```python
from build123d import *

# Parameters (mm, degrees)
SKETCH1_W                 = 55.88
SKETCH1_H                 = 6.35
CUT_EXTRUDE1_START        = -5.588
CUT_EXTRUDE1_DEPTH        = 5.588
CUT_EXTRUDE2_DEPTH        = 5.588
F_8_32_TAPPED_HOLE1_D     = 3.4544
F_8_32_TAPPED_HOLE1_DEPTH = 12.7
F_8_32_TAPPED_HOLE1_TIP   = 1.037806461
F_8_32_TAPPED_HOLE2_D     = 3.4544
F_8_32_TAPPED_HOLE2_DEPTH = 12.7
F_8_32_TAPPED_HOLE2_TIP   = 1.037806461
FILLET1_R                 = 1.5875
CHAMFER1_SIZE             = 0.254
CUT_EXTRUDE3_DEPTH        = 1.5875


with BuildPart() as part:
    # Sketch1 → Revolve1 (revolve)
    with BuildSketch(Plane(origin=(0, 0, 0), x_dir=(0, 0, -1), z_dir=(1, 0, 0)), mode=Mode.PRIVATE) as revolve1_sk:
        with Locations((27.94, 3.175)):
            Rectangle(SKETCH1_W, SKETCH1_H)
    revolve(revolve1_sk.sketch.rotate(Axis((0, 0, 0), (0, 0, -1)), 90), axis=Axis((0, 0, 0), (0, 0, -1)))

    # Sketch5 → Cut-Extrude1 (cut)
    with BuildSketch(Plane.XY.offset(CUT_EXTRUDE1_START)):
        with BuildLine():
            Line((-4.200130206, 4.7625), (4.200130206, 4.7625))
            ThreePointArc((4.200130206, 4.7625), (0, 6.35), (-4.200130206, 4.7625))
        make_face()
        with BuildLine():
            Line((-4.200130206, -4.7625), (4.200130206, -4.7625))
            ThreePointArc((4.200130206, -4.7625), (0, -6.35), (-4.200130206, -4.7625))
        make_face()
    extrude(amount=CUT_EXTRUDE1_DEPTH, mode=Mode.SUBTRACT)

    # Sketch6 → Cut-Extrude2 (cut)
    with BuildSketch(Plane(origin=(0, 0, -55.88), x_dir=(-1, 0, 0), z_dir=(0, 0, -1))):
        with BuildLine():
            Line((-4.200130206, 4.7625), (4.200130206, 4.7625))
            ThreePointArc((4.200130206, 4.7625), (0, 6.35), (-4.200130206, 4.7625))
        make_face()
        with BuildLine():
            Line((4.200130206, -4.7625), (-4.200130206, -4.7625))
            ThreePointArc((-4.200130206, -4.7625), (0, -6.35), (4.200130206, -4.7625))
        make_face()
    extrude(amount=-CUT_EXTRUDE2_DEPTH, mode=Mode.SUBTRACT)

    # #8-32 Tapped Hole1
    with Locations(Plane.XY):
        with Locations((0, 0)):
            Hole(F_8_32_TAPPED_HOLE1_D / 2, depth=F_8_32_TAPPED_HOLE1_DEPTH)
            with Locations((0, 0, -(F_8_32_TAPPED_HOLE1_DEPTH + F_8_32_TAPPED_HOLE1_TIP / 2))):  # 118° drill point
                Cone(0, F_8_32_TAPPED_HOLE1_D / 2, F_8_32_TAPPED_HOLE1_TIP, mode=Mode.SUBTRACT)

    # #8-32 Tapped Hole2
    with Locations(Plane(origin=(0, 0, -55.88), x_dir=(-1, 0, 0), z_dir=(0, 0, -1))):
        with Locations((0, 0)):
            Hole(F_8_32_TAPPED_HOLE2_D / 2, depth=F_8_32_TAPPED_HOLE2_DEPTH)
            with Locations((0, 0, -(F_8_32_TAPPED_HOLE2_DEPTH + F_8_32_TAPPED_HOLE2_TIP / 2))):  # 118° drill point
                Cone(0, F_8_32_TAPPED_HOLE2_D / 2, F_8_32_TAPPED_HOLE2_TIP, mode=Mode.SUBTRACT)

    # Fillet1
    fillet1_edges = [part.edges().sort_by_distance(p)[0] for p in [
        (-4.200130206, 4.7625, -2.794),
        (4.200130206, 4.7625, -2.794),
        (4.200130206, -4.7625, -2.794),
        (-4.200130206, -4.7625, -2.794),
        (4.200130206, 4.7625, -53.086),
        (-4.200130206, 4.7625, -53.086),
        (-4.200130206, -4.7625, -53.086),
        (4.200130206, -4.7625, -53.086),
    ]]
    fillet(fillet1_edges, radius=FILLET1_R)

    # Chamfer1
    chamfer1_edges = [part.edges().sort_by_distance(p)[0] for p in [
        (-6.35, 0, -55.88),
        (5.931994479, -2.26582027, -55.88),
        (-6.35, 0, 0),
        (5.931994479, -2.26582027, 0),
        (0, -4.7625, 0),
        (0, 4.7625, 0),
        (-4.197852075, 4.6241826, 0),
        (4.197852075, 4.6241826, 0),
        (4.197852075, -4.6241826, 0),
        (-4.197852075, -4.6241826, 0),
        (0, -4.7625, -55.88),
        (0, 4.7625, -55.88),
        (4.197852075, 4.6241826, -55.88),
        (-4.197852075, 4.6241826, -55.88),
        (4.197852075, -4.6241826, -55.88),
        (-4.197852075, -4.6241826, -55.88),
    ]]
    chamfer(chamfer1_edges, length=CHAMFER1_SIZE)

    # Sketch11 → Cut-Extrude3 (cut)
    with BuildSketch(Plane(origin=(0, 6.35, 0), x_dir=(-1, 0, 0), z_dir=(0, 1, 0))):
        with BuildLine():
            Line((-1.5875, -34.29), (-1.5875, -21.59))
            ThreePointArc((-1.5875, -21.59), (0, -20.0025), (1.5875, -21.59))
            Line((1.5875, -21.59), (1.5875, -34.29))
            ThreePointArc((1.5875, -34.29), (0, -35.8775), (-1.5875, -34.29))
        make_face()
    extrude(amount=-CUT_EXTRUDE3_DEPTH, mode=Mode.SUBTRACT)


solid = part.part
```
The listing builds one solid part. Answer for the finished solid, in the listing's coordinates (mm). A direction names the side the tool comes from. Give positions to 0.01 mm unless a question says otherwise; leave off trailing zeros. Loops run counter-clockwise (first coordinate to the right, second up) from the corner with the lowest first, then second, coordinate; pieces in that order, holes last. Notation, with made-up numbers: M 58,-12 L 77,-12 A37 ccw 77,26 Z; hole C -19.5,72.25 d5. An arc over 180 degrees is marked long. One line per item, written item: value.
1. Find the intervals of material crossed by probe 1 along Y at (x, z) = (0, -4.5); probe 2 along Y at (x, z) = (0, -45.5); probe 3 along Z at (x, y) = (-1.75, 5.5), in increasing order.
Found:
probe 1: -4.76 to -1.73, 1.73 to 4.76
probe 2: -6.35 to -1.73, 1.73 to 6.35
probe 3: -50.29 to -5.59
2. For a pull along Y with two mould halves and no side action, classify faces 4 (the face through (-0.225, 1.713, -49.441)), 5 (the face through (1.588, 5, -28)), 6 (the face through (-0.138, -0.266, -42.322)), 7 (the face through (-4.21, -4.62, -2.88)) as pulls with the +Y half, pulls with the -Y half, needs draft (parallel to the pull), parting line crosses it, or undercut.
Found:
face 4: undercut
face 5: needs draft
face 6: undercut
face 7: pulls with the -Y half
3. Each of these flat-tipped pins is pushed along its axis until it touches: P1, Ø2, axis at x = 0, y = 0, coming from the -Z side; P2, Ø2, axis at x = 1.5, z = -23.5, coming from the -Y side; P3, Ø2.5, axis at x = 0, z = -26, coming from the +Y side. Where does it stop, or does it pass through?
Found:
P1: z = -42.74
P2: y = -6.33
P3: y = 4.76
4. For faces 1 (the face through (-0.035, 5.568, -35.877)), 2 (the face through (0, -4.762, -53)), 3 (the face through (-4.21, 4.62, -52.92)), determine the directions among +Z, -Z, +X, -X, +Y, -Y from which every point of the face is accessible in a straight line to the end or side of a thin tool.
Found:
face 1: +Y
face 2: -Z, +X, -X, -Y
face 3: -Z, -X, +Y
5. Section B-B on x = -3 is taken. Determine the outline of the cut face in (y, z).
Found:
outline: M -5.6,-50.29 L -4.76,-50.29 L -4.76,-55.63 L -4.51,-55.88 L 4.51,-55.88 L 4.76,-55.63 L 4.76,-50.29 L 5.6,-50.29 L 5.6,-5.59 L 4.76,-5.59 L 4.76,-0.25 L 4.51,0 L -4.51,0 L -4.76,-0.25 L -4.76,-5.59 L -5.6,-5.59 Z
6. Section A-A on z = -29 is taken. Determine the outline of the cut face in (x, y).
Found:
outline: M -1.59,4.76 L -1.59,6.15 A6.35 ccw long 1.59,6.15 L 1.59,4.76 Z
7. Section C-C on z = -38.5 is taken. Determine the outline of the cut face in (x, y).
Found:
outline: C 0,0 d12.7
